Model file for the job. Use its own axes, mm. A direction names the side the tool comes from. Give positions to 0.01 mm unless a question says otherwise; leave off trailing zeros. Write each loop counter-clockwise with the first axis right and the second up, starting at its lowest first coordinate (ties: lowest second). Pieces come first, ordered by that corner, then holes.
```python
from build123d import *

# Parameters (mm, degrees)
SKETCH1_W           = 25.4
SKETCH1_H           = 50.8
BOSS_EXTRUDE1_DEPTH = 279.4
SHELL1_T            = -3.175
SKETCH3_R           = 2.38125
CUT_EXTRUDE1_DEPTH  = 285.264471927


with BuildPart() as part:
    # Sketch1 → Boss-Extrude1 (new, symmetric)
    with BuildSketch(Plane.XY):
        Rectangle(SKETCH1_W, SKETCH1_H)
    extrude(amount=BOSS_EXTRUDE1_DEPTH, both=True)

    # Shell1
    shell1_openings = [part.faces().sort_by_distance(p)[0] for p in [
        (0, 0, 279.4),
        (0, 0, -279.4),
    ]]
    offset(amount=SHELL1_T, openings=shell1_openings, kind=Kind.INTERSECTION)

    # Sketch3 → Cut-Extrude1 (cut, through all)
    with BuildSketch(Plane(origin=(0, 25.4, 0), x_dir=(1, 0, 0), z_dir=(0, 1, 0))):
        with Locations(Location((0, 266.7, 0), (0, 0, 270))):
            Circle(SKETCH3_R)
        with Locations(Location((0, 241.3, 0), (0, 0, 270))):
            Circle(SKETCH3_R)
        with Locations(Location((0, 215.9, 0), (0, 0, 270))):
            Circle(SKETCH3_R)
        with Locations(Location((0, -215.9, 0), (0, 0, 270))):
            Circle(SKETCH3_R)
        with Locations(Location((0, -241.3, 0), (0, 0, 270))):
            Circle(SKETCH3_R)
        with Locations(Location((0, -266.7, 0), (0, 0, 270))):
            Circle(SKETCH3_R)
        with BuildLine():
            Line((6.35, 279.4), (-12.7, 279.4))
            Line((-12.7, 279.4), (-12.7, 273.05))
            Line((-12.7, 273.05), (0, 273.05))
            ThreePointArc((0, 273.05), (4.490128061, 274.909871939), (6.35, 279.4))
        make_face()
        with BuildLine():
            Line((-12.7, -273.05), (0, -273.05))
            ThreePointArc((0, -273.05), (4.490128061, -274.909871939), (6.35, -279.4))
            Line((6.35, -279.4), (-12.7, -279.4))
            Line((-12.7, -279.4), (-12.7, -273.05))
        make_face()
    extrude(amount=-CUT_EXTRUDE1_DEPTH, mode=Mode.SUBTRACT)


solid = part.part
```
1. Which spindle directions (+Z, -Z, +X, -X, +Y, -Y) get a long thin tool onto all of the face, cutting with end or side? Do faces 1 (the flat face through (-10, -2, 273.05)), 2 (the flat face through (-10, -2, -273.05)), 3 (the flat face through (12.7, 0, 4)), 4 (the flat face through (9.525, 0, 4)). Say none if no direction does.
Calculated:
face 1: +Z, -X, +Y, -Y
face 2: -Z, -X, +Y, -Y
face 3: +Z, -Z, +X, +Y, -Y
face 4: +Z, -Z
2. Pull direction Y, two halves, no side cores. Call faces 5 (the flat face through (-9.525, 0, 4)), 6 (the flat face through (0, -25.4, 4)), 7 (the flat face through (0, -22.225, 4)), 8 (the flat face through (-12.7, 0, 4)): +Y half, -Y half, draft (parallel to the pull), parting line (faces both ways), or undercut.
Calculated:
face 5: undercut
face 6: -Y half
face 7: undercut
face 8: draft
3. Pin check, flat tip, straight feed: P1, Ø3, axis at x = 0, z = 266.7, coming from the -Y side. Stop position of the tip, or through.
Calculated:
P1: passes through
4. Probe probe 1 along X at (y, z) = (-23, 241); probe 2 along Y at (x, z) = (-0.5, -87) (3 decimals); probe 3 along X at (y, z) = (-5.5, -243.5) (3 decimals). List the from-to ranges inside material, lowest first.
Calculated:
probe 1: x = -12.7 to -2.36, 2.36 to 12.7
probe 2: y = -25.4 to -22.225, 22.225 to 25.4
probe 3: x = -12.7 to -9.525, 9.525 to 12.7
5. Slice it at B-B, the plane z = 153. Write the cut outline in (x, y) (3 decimals).
Calculated:
outline: (-12.7, -25.4) - (12.7, -25.4) - (12.7, 25.4) - (-12.7, 25.4) - close; hole (-9.525, -22.225) - (9.525, -22.225) - (9.525, 22.225) - (-9.525, 22.225) - close
6. Slice it at A-A, the plane y = 13.5. Write the cut outline in (x, z) (3 decimals).
Calculated:
outline: (-12.7, -273.05) - (-9.525, -273.05) - (-9.525, 273.05) - (-12.7, 273.05) - close; (9.525, -279.4) - (12.7, -279.4) - (12.7, 279.4) - (9.525, 279.4) - close
